Autodesk Inventor part; units mm, degrees
ref_plane "YZ Plane" through (0, 0, 0) normal (1, 0, 0) x (0, 1, 0)
ref_plane "XZ Plane" through (0, 0, 0) normal (0, 1, 0) x (-1, 0, 0)
ref_plane "XY Plane" through (0, 0, 0) normal (0, 0, 1) x (1, 0, 0)
sketch "Sketch1" plane through (0, 0, 0) normal (0, 0, 1) x (1, 0, 0)
  line L0 (57.983, -13.2177) -> (41.983, -13.2177)
  line L1 (41.983, -18.2177) -> (57.983, -18.2177)
  line L2 (-58.017, -13.2177) -> (-42.017, -13.2177)
  line L3 (-42.017, -18.2177) -> (-58.017, -18.2177)
  line L4 (32.983, -13.2177) -> (-33.017, -13.2177)
  line L5 (-33.017, -18.2177) -> (32.983, -18.2177)
  arc A0 (34.983, -15.2177) -> (32.983, -13.2177) centre (32.983, -15.2177) ccw
  arc A1 (-35.017, -16.2177) -> (-33.017, -18.2177) centre (-33.017, -16.2177) ccw
  arc A2 (-33.017, -13.2177) -> (-35.017, -15.2177) centre (-33.017, -15.2177) ccw
  arc A3 (-40.017, -15.2177) -> (-42.017, -13.2177) centre (-42.017, -15.2177) ccw
  arc A4 (-42.017, -18.2177) -> (-40.017, -16.2177) centre (-42.017, -16.2177) ccw
  arc A5 (-60.017, -16.2177) -> (-58.017, -18.2177) centre (-58.017, -16.2177) ccw
  arc A6 (-58.017, -13.2177) -> (-60.017, -15.2177) centre (-58.017, -15.2177) ccw
  arc A7 (39.983, -16.2177) -> (41.983, -18.2177) centre (41.983, -16.2177) ccw
  arc A8 (41.983, -13.2177) -> (39.983, -15.2177) centre (41.983, -15.2177) ccw
  arc A9 (59.983, -15.2177) -> (57.983, -13.2177) centre (57.983, -15.2177) ccw
  arc A10 (57.983, -18.2177) -> (59.983, -16.2177) centre (57.983, -16.2177) ccw
  arc A11 (32.983, -18.2177) -> (34.983, -16.2177) centre (32.983, -16.2177) ccw
  line L6 (59.983, -15.2177) -> (39.983, -15.2177)
  line L7 (39.983, -16.2177) -> (59.983, -16.2177)
  line L8 (34.983, -15.2177) -> (-35.017, -15.2177)
  line L9 (-35.017, -16.2177) -> (34.983, -16.2177)
  line L10 (-40.017, -15.2177) -> (-60.017, -15.2177)
  line L11 (-60.017, -16.2177) -> (-40.017, -16.2177)
  line L12 (-57.517, -25.0011) -> (-110.517, -25.0011)
  line L13 (-110.517, -25.0011) -> (-110.517, -20.0011)
  line L14 (-57.517, -20.0011) -> (-110.517, -20.0011)
  line L15 (-57.517, -25.0011) -> (-57.517, -20.0011)
  line L16 (-140.517, -25.0011) -> (-195.517, -25.0011)
  line L17 (-195.517, -25.0011) -> (-195.517, -20.0011)
  line L18 (-140.517, -20.0011) -> (-195.517, -20.0011)
  line L19 (-140.517, -25.0011) -> (-140.517, -20.0011)
  line L20 (-225.517, -25.0011) -> (-255.517, -25.0011)
  line L21 (-255.517, -25.0011) -> (-255.517, -20.0011)
  line L22 (-225.517, -20.0011) -> (-255.517, -20.0011)
  line L23 (-225.517, -25.0011) -> (-225.517, -20.0011)
  line L24 (-272.017, -33.0013) -> (103.983, -33.0013)
  line L25 (98.983, 19.9989) -> (98.983, 9.9974)
  line L26 (98.983, 9.9974) -> (93.983, 9.9974)
  line L27 (93.983, 19.9989) -> (93.983, 9.9974)
  line L28 (98.983, 19.9989) -> (93.983, 19.9989)
  line L29 (98.983, -10.0026) -> (98.983, -25.0018)
  line L30 (98.983, -25.0018) -> (93.983, -25.0018)
  line L31 (93.983, -10.0026) -> (93.983, -25.0018)
  line L32 (98.983, -10.0026) -> (93.983, -10.0026)
  line L33 (-262.017, -10.0026) -> (-262.017, -25.0018)
  line L34 (-262.017, -25.0018) -> (-267.017, -25.0018)
  line L35 (-267.017, -10.0026) -> (-267.017, -25.0018)
  line L36 (-262.017, -10.0026) -> (-267.017, -10.0026)
  line L37 (-262.017, 19.9989) -> (-262.017, 9.9974)
  line L38 (-262.017, 9.9974) -> (-267.017, 9.9974)
  line L39 (-267.017, 19.9989) -> (-267.017, 9.9974)
  line L40 (-262.017, 19.9989) -> (-267.017, 19.9989)
  line L41 (-110.017, -13.2177) -> (-126.017, -13.2177)
  line L42 (-126.017, -18.2177) -> (-110.017, -18.2177)
  line L43 (-226.017, -13.2177) -> (-210.017, -13.2177)
  line L44 (-210.017, -18.2177) -> (-226.017, -18.2177)
  line L45 (-135.017, -13.2177) -> (-201.017, -13.2177)
  line L46 (-201.017, -18.2177) -> (-135.017, -18.2177)
  arc A12 (-133.017, -15.2177) -> (-135.017, -13.2177) centre (-135.017, -15.2177) ccw
  arc A13 (-203.017, -16.2177) -> (-201.017, -18.2177) centre (-201.017, -16.2177) ccw
  arc A14 (-201.017, -13.2177) -> (-203.017, -15.2177) centre (-201.017, -15.2177) ccw
  arc A15 (-208.017, -15.2177) -> (-210.017, -13.2177) centre (-210.017, -15.2177) ccw
  arc A16 (-210.017, -18.2177) -> (-208.017, -16.2177) centre (-210.017, -16.2177) ccw
  arc A17 (-228.017, -16.2177) -> (-226.017, -18.2177) centre (-226.017, -16.2177) ccw
  arc A18 (-226.017, -13.2177) -> (-228.017, -15.2177) centre (-226.017, -15.2177) ccw
  arc A19 (-128.017, -16.2177) -> (-126.017, -18.2177) centre (-126.017, -16.2177) ccw
  arc A20 (-126.017, -13.2177) -> (-128.017, -15.2177) centre (-126.017, -15.2177) ccw
  arc A21 (-108.017, -15.2177) -> (-110.017, -13.2177) centre (-110.017, -15.2177) ccw
  arc A22 (-110.017, -18.2177) -> (-108.017, -16.2177) centre (-110.017, -16.2177) ccw
  arc A23 (-135.017, -18.2177) -> (-133.017, -16.2177) centre (-135.017, -16.2177) ccw
  line L47 (-108.017, -15.2177) -> (-128.017, -15.2177)
  line L48 (-128.017, -16.2177) -> (-108.017, -16.2177)
  line L49 (-133.017, -15.2177) -> (-203.017, -15.2177)
  line L50 (-203.017, -16.2177) -> (-133.017, -16.2177)
  line L51 (-208.017, -15.2177) -> (-228.017, -15.2177)
  line L52 (-228.017, -16.2177) -> (-208.017, -16.2177)
  line L53 (87.483, -25.0011) -> (57.483, -25.0011)
  line L54 (57.483, -25.0011) -> (57.483, -20.0011)
  line L55 (87.483, -20.0011) -> (57.483, -20.0011)
  line L56 (87.483, -25.0011) -> (87.483, -20.0011)
  line L57 (27.483, -25.0011) -> (-27.517, -25.0011)
  line L58 (-27.517, -25.0011) -> (-27.517, -20.0011)
  line L59 (27.483, -20.0011) -> (-27.517, -20.0011)
  line L60 (27.483, -25.0011) -> (27.483, -20.0011)
  circle A24 centre (-84.017, -1.0005) radius 3
  line L61 (103.983, 20.9995) -> (103.983, -33.0013)
  circle A25 centre (-0.017, -1.0005) radius 3
  line L62 (-272.017, 20.9995) -> (-272.017, -33.0013)
  circle A26 centre (-168.017, -1.0005) radius 3
  line L63 (101.983, 22.9995) -> (-270.017, 22.9995)
  arc A27 (103.983, 20.9995) -> (101.983, 22.9995) centre (101.983, 20.9995) ccw
  arc A28 (-270.017, 22.9995) -> (-272.017, 20.9995) centre (-270.017, 20.9995) ccw
  point P0 (103.983, 22.9995)
  point P1 (59.983, -13.2177)
  point P2 (59.983, -18.2177)
  point P3 (59.983, -16.2177)
  point P4 (-108.017, -13.2177)
  point P5 (-108.017, -18.2177)
  point P6 (-272.017, 22.9995)
  dimension "d17" = 5
  dimension "d27" = 2
  dimension "d36" = 5
  dimension "d37" = 2
  dimension "d39" = 6
  dimension "d40" = 6
  dimension "d42" = 188
  dimension "d44" = 376
  dimension "d45" = 188
  dimension "d46" = 84
  dimension "d47" = 6
  dimension "d48" = 84
  dimension "d50" = 2
extrude "Extrusion1" add sketch "Sketch1" along normal blind 5
properties part number "case top front" material "ABS Plastic"
Geometry check sheet. Reference: the model listing, model coordinates, mm. Round coordinates to 2 decimals unless told otherwise and drop trailing zeros. Loops run counter-clockwise (first coordinate to the right, second up) from the corner with the lowest first, then second, coordinate; pieces in that order, holes last. Notation, with made-up numbers: (64, -22) - (120, -22) arc R12 cw to (120, -10) - close; hole circle Ø10 at (-12.75, 54). An arc over 180 degrees is marked (long way). Write each question's results on one line, items separated by ' | '. Start each with the question number.
Q1. Cross-section at A-A on y = 15.5. Enter the section's corners in (x, z), and give its area (3 significant figures).
Q2. Cross-section at B-B on x = -93.5. Enter the section's corners in (y, z), and give its area (3 significant figures).
Q3. Cross-section at C-C on x = -9.5. Enter the section's corners in (y, z).
Q4. Cross-section at D-D on z = 1. State how many separate pieces and enclosed holes the cut face has, and give its area (3 significant figures).
Q5. Release check for a two-part mould opening along X. For faces 1 (the cylindrical face through (1.596, -3.53, 2.465)), 2 (the flat face through (-87, -5, 5)) record: +X half, -X half, draft (parallel to the pull), parting line (faces both ways), or undercut.
Q6. Thickness scan on line 1 (X direction, y = 11, z = 4.25); line 2 (Y direction, x = -177, z = 3.2); line 3 (Y direction, x = -213, z = 2.65). Record the ranges inside material, lowest first. Write a range as [from, to].
Answers below:
1) outline: (-272.02, 0) - (-267.02, 0) - (-267.02, 5) - (-272.02, 5) - close; (-262.02, 0) - (93.98, 0) - (93.98, 5) - (-262.02, 5) - close; (98.98, 0) - (103.98, 0) - (103.98, 5) - (98.98, 5) - close | area: 1,830 mm²
2) outline: (-33, 0) - (-25, 0) - (-25, 5) - (-33, 5) - close; (-20, 0) - (23, 0) - (23, 5) - (-20, 5) - close | area: 255 mm²
3) outline: (-33, 0) - (-25, 0) - (-25, 5) - (-33, 5) - close; (-20, 0) - (-18.22, 0) - (-18.22, 5) - (-20, 5) - close; (-16.22, 0) - (-15.22, 0) - (-15.22, 5) - (-16.22, 5) - close; (-13.22, 0) - (23, 0) - (23, 5) - (-13.22, 5) - close
4) separate pieces: 1 | enclosed holes: 24 | area: 18,700 mm²
5) face 1: undercut | face 2: draft
6) line 1: x = [-272.02, -267.02], [-262.02, 93.98], [98.98, 103.98] | line 2: y = [-33, -25], [-20, -18.22], [-16.22, -15.22], [-13.22, 23] | line 3: y = [-33, -18.22], [-16.22, -15.22], [-13.22, 23]
